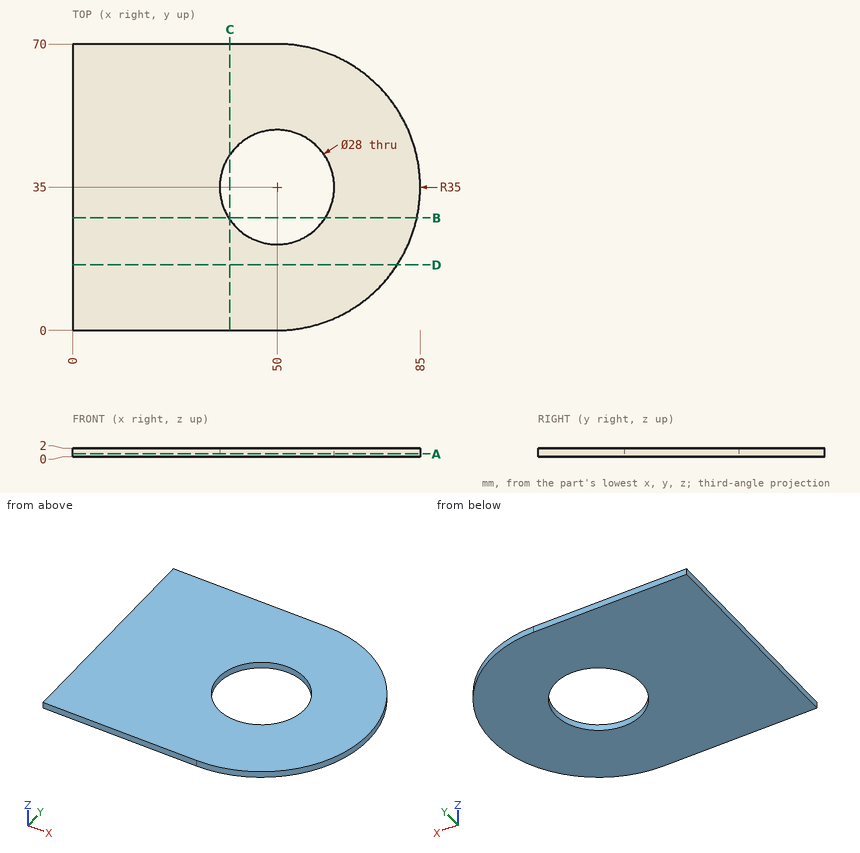
Here's the drawing with two shaded views (mm, measured from the low corner). I have some questions. Coordinates: 2 decimals unless noted, no trailing zeros. Order: outer loops, then holes, each group sorted by start corner. A loop starts at its lowest first (then second) coordinate and runs counter-clockwise, first axis right, second up. Notation, with made-up numbers: (-1.5, -12.75) -> (20.5, -12.75) arc R16 ccw to (20.5, -8.75) -> close; hole circle Ø2 at (-30.5, 68). An arc over 180 degrees is marked (long way). One line per question, with ' | ' between items.
Q1. I'm going to push a flat-ended pin straight in: P1, Ø8, axis at x = 45.5, y = 25.5, coming from the +Z side. Where does the tip first touch, or does it pass through?
Return value:
P1: z = 2
Q2. Imagine slicing it at B-B on y = 27.5. Please give me the cut outline in (x, z), and give its area (3 significant figures).
Return value:
outline: (0, 0) -> (38.18, 0) -> (38.18, 2) -> (0, 2) -> close; (61.82, 0) -> (84.19, 0) -> (84.19, 2) -> (61.82, 2) -> close | area: 121 mm²
Q3. Imagine slicing it at A-A on z = 0.65. Please give me the cut outline in (x, y), and give its area (3 significant figures).
Return value:
outline: (0, 0) -> (50, 0) arc R35 ccw to (50, 70) -> (0, 70) -> close; hole circle Ø28 at (50, 35) | area: 4,810 mm²
Q4. Imagine slicing it at C-C on x = 38.5. Please give me the cut outline in (y, z).
Return value:
outline: (0, 0) -> (27.02, 0) -> (27.02, 2) -> (0, 2) -> close; (42.98, 0) -> (70, 0) -> (70, 2) -> (42.98, 2) -> close
Q5. If I drill on L1, parallel to Y at x = 50, z = 1.05; L2, parallel to X at y = 23.5, z = 1.6; L3, parallel to Y at x = 60, z = 1.65, over which ranges is the centre line in solid material (lowest first)?
Return value:
L1: 0 to 21, 49 to 70 | L2: 0 to 42.02, 57.98 to 83.06 | L3: 1.46 to 25.2, 44.8 to 68.54
Q6. Imagine slicing it at D-D on y = 16. Please give me the cut outline in (x, z).
Return value:
outline: (0, 0) -> (79.39, 0) -> (79.39, 2) -> (0, 2) -> close
